Part model, mm, in its own coordinate system. A direction names the side the tool comes from. Coordinates: 2 decimals unless noted, no trailing zeros. Write each loop counter-clockwise with the first axis right and the second up, starting at its lowest first coordinate (ties: lowest second). Pieces come first, ordered by that corner, then holes. Notation, with made-up numbers: (-40, 33.25) - (18, 33.25) arc R20 ccw to (18, 64.25) - close; hole circle Ø2 at (68, 33). An arc over 180 degrees is marked (long way). Use a Markdown table: item, result.
```python
from build123d import *


with BuildPart() as part:
    # Sketch1 → Revolve1 (revolve)
    with BuildSketch(Plane.XY):
        Polygon((3, -21.375), (11, -21.375), (11, -20.375), (4, -20.375), (4, -18.875), (11, -18.875), (11, -17.875), (4, -17.875), (4, -16.375), (11, -16.375), (11, -15.375), (4, -15.375), (4, -13.875), (11, -13.875), (11, -12.875), (4, -12.875), (4, -11.375), (11, -11.375), (11, -10.375), (4, -10.375), (4, -8.875), (11, -8.875), (11, -7.875), (4, -7.875), (4, -6.375), (11, -6.375), (11, -5.375), (4, -5.375), (4, -3.875), (11, -3.875), (11, -2.875), (4, -2.875), (4, -1.375), (11, -1.375), (11, -0.375), (4, -0.375), (4, 1.125), (11, 1.125), (11, 2.125), (4, 2.125), (4, 3.625), (11, 3.625), (11, 4.625), (4, 4.625), (4, 6.125), (8, 6.125), (8, 7.125), (4, 7.125), (4, 8.625), (8, 8.625), (8, 11.625), (6, 11.625), (6, 17.625), (8, 17.625), (8, 21.375), (4.8641, 21.375), (4.8641, 11.375), (2, 6.414233282), (2, 2.414233282), (1, 1.836883013), (1, -5.895299462), (3, -7.05), align=None)
    revolve(axis=Axis((0, -21.375, 0), (0, 1, 0)))


solid = part.part
```
Item 1: Drill centre lines: probe 1 along Z at (x, y) = (0, 14.75); probe 2 along X at (y, z) = (-12.25, 0). Where is each one in solid material? Low to high.
From the geometry:
| item | result |
|---|---|
| probe 1 | -6 to -4.86, 4.86 to 6 |
| probe 2 | -4 to -3, 3 to 4 |
Item 2: Two-plate mould, pull along Y, no slides. Class faces 1 (the face through (-0.1, 21.375, 5.2)), 2 (the face through (-2.38, 4.13, 10.74)), 3 (the face through (0, -2.875, 5)): pulls with the +Y half, pulls with the -Y half, needs draft (parallel to the pull), parting line crosses it, or undercut.
From the geometry:
| item | result |
|---|---|
| face 1 | pulls with the +Y half |
| face 2 | needs draft |
| face 3 | undercut |
Item 3: Which spindle directions (+Z, -Z, +X, -X, +Y, -Y) get a long thin tool onto all of the face, cutting with end or side? Do faces 4 (the face through (-1.05, 16.3, 4.75)), 5 (the face through (0, -7.875, 5)), 6 (the face through (-2.38, -3.37, 10.74)). Say none if no direction does.
From the geometry:
| item | result |
|---|---|
| face 4 | +Y |
| face 5 | none |
| face 6 | +Y, -Y |
Item 4: Band-saw the part on A-A, the plane y = -4.5. Give the cut face in (x, z), then the cut area to 3 significant figures.
From the geometry:
| item | result |
|---|---|
| outline | circle Ø8 at (0, 0); hole circle Ø2 at (0, 0) |
| area | 47.1 mm^2 |
Item 5: Drop flat-ended pins along their axis: P1, Ø11, axis at x = 0.5, z = 4.5, coming from the +Y side (3 decimals); P2, Ø1.5, axis at y = -7, z = -3, coming from the +X side; P3, Ø2, axis at y = -16, z = -7, coming from the -X side; P4, Ø1, axis at x = -3, y = 5.5, coming from the -Z side. Give the stop position or say it passes through.
From the geometry:
| item | result |
|---|---|
| P1 | y = 21.375 |
| P2 | x = 10.69 |
| P3 | x = -9.22 |
| P4 | z = -3.12 |
Item 6: Band-saw the part on B-B, the plane z = 7.25. Count the separate pieces of the cut face and the enclosed holes in it, then the cut area to 3 significant figures.
From the geometry:
| item | result |
|---|---|
| separate pieces | 14 |
| enclosed holes | 0 |
| area | 234 mm^2 |
Item 7: Band-saw the part on D-D, the plane y = 12.5. Give the cut face in (x, z).
From the geometry:
| item | result |
|---|---|
| outline | circle Ø12 at (0, 0); hole circle Ø9.73 at (0, 0) |
